from build123d import *

# Parameters (mm, degrees)
SKETCH3_W                                        = 25.4
SKETCH3_H                                        = 7.9375
BOSS_EXTRUDE1_DEPTH                              = 24
CSK_FOR_1_4_FLAT_HEAD_MACHINE_SCREW1_D           = 6.7564
CSK_FOR_1_4_FLAT_HEAD_MACHINE_SCREW1_CSINK_D     = 12.8778
CSK_FOR_1_4_FLAT_HEAD_MACHINE_SCREW1_CSINK_ANGLE = 82


with BuildPart() as part:
    # Sketch3 → Boss-Extrude1 (new body, symmetric)
    with BuildSketch(Plane.XY):
        Rectangle(SKETCH3_W, SKETCH3_H)
    extrude(amount=BOSS_EXTRUDE1_DEPTH, both=True)

    # CSK for 1/4 Flat Head Machine Screw1 (through all)
    with Locations(Plane(origin=(0, 3.96875, 0), x_dir=(-1, 0, 0), z_dir=(0, 1, 0))):
        with Locations((0, 14.1), (0, -11.3)):
            CounterSinkHole(CSK_FOR_1_4_FLAT_HEAD_MACHINE_SCREW1_D / 2, CSK_FOR_1_4_FLAT_HEAD_MACHINE_SCREW1_CSINK_D / 2, counter_sink_angle=CSK_FOR_1_4_FLAT_HEAD_MACHINE_SCREW1_CSINK_ANGLE)


solid = part.part
Check sheet for the modelled part. Datum: model origin and axes. Units: mm. Coordinates: 2 decimals unless noted, no trailing zeros. Loops run counter-clockwise (first coordinate to the right, second up) from the corner with the lowest first, then second, coordinate; pieces in that order, holes last. Notation, with made-up numbers: (46.5, 3) -> (96.5, 3) arc R12 ccw to (96.5, 12) -> close; hole circle Ø4 at (3.5, 89). An arc over 180 degrees is marked (long way). Answer in a Markdown table with one row per item.
1. Material ranges on line 1 along Z through (x, y) = (0, -2.35); line 2 along X through (y, z) = (-0.85, -11.3); line 3 along Z through (x, y) = (2.5, 0.5), recorded low to high. Write a range as [from, to].
Check values:
| item | result |
|---|---|
| line 1 | z = [-24, -14.68], [-7.92, 10.72], [17.48, 24] |
| line 2 | x = [-12.7, -3.38], [3.38, 12.7] |
| line 3 | z = [-24, -13.64], [-8.96, 11.76], [16.44, 24] |
2. Sectioned sample at C-C, the plane y = -0.5. Record the boundary of the cut face in (x, z), then the cut area to 3 significant figures.
Check values:
| item | result |
|---|---|
| outline | (-12.7, -24) -> (12.7, -24) -> (12.7, 24) -> (-12.7, 24) -> close; hole circle Ø6.76 at (0, -11.3); hole circle Ø6.76 at (0, 14.1) |
| area | 1,150 mm2 |
3. Go/stop test with flat-tipped pins: pin 1 (8 mm diameter, centred on x = 0, z = 14.1, fed in from +Y); pin 2 (11 mm diameter, centred on x = 0, z = -11.3, fed in from -Y). Record where each tip stops, or that it passes through.
Check values:
| item | result |
|---|---|
| pin 1 | stops at y = 1.16 |
| pin 2 | stops at y = -3.97 |
4. Sectioned sample at A-A, the plane x = 0. Record the boundary of the cut face in (y, z), then the cut area to 3 significant figures.
Check values:
| item | result |
|---|---|
| outline | (-3.97, -24) -> (3.97, -24) -> (3.97, -17.74) -> (0.45, -14.68) -> (-3.97, -14.68) -> close; (-3.97, -7.92) -> (0.45, -7.92) -> (3.97, -4.86) -> (3.97, 7.66) -> (0.45, 10.72) -> (-3.97, 10.72) -> close; (-3.97, 17.48) -> (0.45, 17.48) -> (3.97, 20.54) -> (3.97, 24) -> (-3.97, 24) -> close |
| area | 252 mm2 |
5. Release check for a two-part mould opening along X. For faces 1 (the face through (12.7, 0, 0)), 2 (the face through (-0.44, -1.79, -7.95)), 3 (the face through (-2.8, 0.62, -13.45)), 4 (the face through (0, 0, 24)) record: released by +X, released by -X, zero draft, split by the parting line, or undercut.
Check values:
| item | result |
|---|---|
| face 1 | released by +X |
| face 2 | undercut |
| face 3 | undercut |
| face 4 | zero draft |
6. Sectioned sample at B-B, the plane z = -11.3. Record the boundary of the cut face in (x, y), then the cut area to 3 significant figures.
Check values:
| item | result |
|---|---|
| outline | (-12.7, -3.97) -> (-3.38, -3.97) -> (-3.38, 0.45) -> (-6.44, 3.97) -> (-12.7, 3.97) -> close; (3.38, -3.97) -> (12.7, -3.97) -> (12.7, 3.97) -> (6.44, 3.97) -> (3.38, 0.45) -> close |
| area | 137 mm2 |
7. Sectioned sample at D-D, the plane y = 3. Record the boundary of the cut face in (x, z), then the cut area to 3 significant figures.
Check values:
| item | result |
|---|---|
| outline | (-12.7, -24) -> (12.7, -24) -> (12.7, 24) -> (-12.7, 24) -> close; hole circle Ø11.19 at (0, -11.3); hole circle Ø11.19 at (0, 14.1) |
| area | 1,020 mm2 |
